For this review, take the finished solid that the model builds, in its own axes (mm). A direction names the side the tool comes from. Coordinates: 2 decimals unless noted, no trailing zeros. Write each loop counter-clockwise with the first axis right and the second up, starting at its lowest first coordinate (ties: lowest second). Pieces come first, ordered by that corner, then holes. Notation, with made-up numbers: M -0.75,12 L 26.25,12 A17 cw 26.25,26 Z; hole C -32,53.25 d2. An arc over 180 degrees is marked long. Return JSON: item names as keys, results as strings.
```python
from build123d import *
from build123d.topology import SkipClean

# Parameters (mm, degrees)
BOSS_EXTRUDE1_DEPTH = 2.032
SKETCH2_R           = 3.81
SKETCH2_R_2         = 1.143
CUT_EXTRUDE1_DEPTH  = 13.861532724
BOSS_EXTRUDE2_START = 9.652
SKETCH3_R           = 7.62
SKETCH3_R_2         = 6.82
BOSS_EXTRUDE2_DEPTH = 9.652
SKETCH4_W           = 25.828848912
SKETCH4_H           = 4.572
CUT_EXTRUDE2_DEPTH  = 16.951523564
BOSS_EXTRUDE3_START = 11.43
SKETCH5_R           = 6.82
BOSS_EXTRUDE3_DEPTH = 11.43


with BuildPart() as part:
    # Sketch1 → Boss-Extrude1 (new body)
    with BuildSketch(Plane(origin=(0, 0, 0), x_dir=(1, 0, 0), z_dir=(0, 1, 0))):
        with BuildLine():
            ThreePointArc((-6.530513036, -3.926423243), (0, -7.62), (6.530513036, -3.926423243))
            ThreePointArc((6.530513036, -3.926423243), (7.220592933, -3.152220394), (8.145517241, -2.683055883))
            ThreePointArc((8.145517241, -2.683055883), (10.16, 0), (8.145517241, 2.683055883))
            ThreePointArc((8.145517241, 2.683055883), (7.220592933, 3.152220394), (6.530513036, 3.926423243))
            ThreePointArc((6.530513036, 3.926423243), (0, 7.62), (-6.530513036, 3.926423243))
            ThreePointArc((-6.530513036, 3.926423243), (-7.220592933, 3.152220394), (-8.145517241, 2.683055883))
            ThreePointArc((-8.145517241, 2.683055883), (-10.16, 0), (-8.145517241, -2.683055883))
            ThreePointArc((-8.145517241, -2.683055883), (-7.220592933, -3.152220394), (-6.530513036, -3.926423243))
        make_face()
    extrude(amount=BOSS_EXTRUDE1_DEPTH)

    # Sketch2 → Cut-Extrude1 (cut, through all)
    with BuildSketch(Plane(origin=(0, 2.032, 0), x_dir=(1, 0, 0), z_dir=(0, 1, 0))):
        with Locations(Location((0, 0, 0), (0, 0, 270))):
            Circle(SKETCH2_R)
        with Locations(Location((-7.366, 0, 0), (0, 0, 270))):
            Circle(SKETCH2_R_2)
        with Locations(Location((7.366, 0, 0), (0, 0, 270))):
            Circle(SKETCH2_R_2)
    extrude(amount=-CUT_EXTRUDE1_DEPTH, mode=Mode.SUBTRACT)

    # Sketch3 → Boss-Extrude2 (add)
    with SkipClean():  # the faces are left unmerged after this step: merging them gives an invalid solid
        with BuildSketch(Plane.XZ.offset(BOSS_EXTRUDE2_START)):
            with Locations(Location((0, 0, 0), (0, 0, 270))):
                Circle(SKETCH3_R)
            with Locations(Location((0, 0, 0), (0, 0, 171.875802718))):
                Circle(SKETCH3_R_2, mode=Mode.SUBTRACT)
        extrude(amount=-BOSS_EXTRUDE2_DEPTH)

    # Sketch4 → Cut-Extrude2 (cut, through all)
    with SkipClean():  # the faces are left unmerged after this step: merging them gives an invalid solid
        with BuildSketch(Plane.XZ):
            Rectangle(SKETCH4_W, SKETCH4_H)
        extrude(amount=CUT_EXTRUDE2_DEPTH, mode=Mode.SUBTRACT)

    # Sketch5 → Boss-Extrude3 (add)
    with SkipClean():  # the faces are left unmerged after this step: merging them gives an invalid solid
        with BuildSketch(Plane.XZ.offset(BOSS_EXTRUDE3_START)):
            with Locations(Location((0, 0, 0), (0, 0, 160.415870392))):
                Circle(SKETCH5_R)
        extrude(amount=-BOSS_EXTRUDE3_DEPTH)


solid = part.part
```
1. Clearance check with flat-ended pins moving along their axes: pin 1 Ø1 at (x, y) = (5, -3.5) entering from -Z; pin 2 Ø2 at (y, z) = (-9.5, -4) entering from +X; pin 3 Ø8 at (y, z) = (0.5, 5) entering from +X. State where each tip first meets the part, or that it passes through.
Checks:
{"pin 1": "z = -6.15", "pin 2": "x = 7", "pin 3": "x = 9.97"}
2. Draft analysis for pull direction X (two halves, no side actions). For faces 1 (the face through (-0.14, -3.89, -7.62)), 2 (the face through (6.25, 1.03, -0.25)), 3 (the face through (7, -5, 2.286)), 4 (the face through (3.778, 1.03, -0.496)), state which applies: +X half, -X half, draft (parallel to the pull), parting line (faces both ways), or undercut.
Checks:
{"face 1": "parting line", "face 2": "undercut", "face 3": "draft", "face 4": "undercut"}
3. We need section C-C (y = -5). State the section outline as (x, z) points.
Checks:
{"outline": "M -7.27,-2.29 A7.62 ccw 7.27,-2.29 L 6.43,-2.29 A6.82 ccw 6.43,2.29 L 7.27,2.29 A7.62 ccw -7.27,2.29 L -6.43,2.29 A6.82 ccw -6.43,-2.29 Z"}
4. We need section D-D (z = -3). State the section outline as (x, y) points.
Checks:
{"outline": "M -7.44,0 L -7,0 L -7,-9.65 L -6.12,-9.65 L -6.12,-11.43 L 6.12,-11.43 L 6.12,-9.65 L 7,-9.65 L 7,0 L 7.44,0 L 7.44,2.03 L 2.35,2.03 L 2.35,0 L -2.35,0 L -2.35,2.03 L -7.44,2.03 Z"}
5. We need section A-A (x = 0). State the section outline as (y, z) points, plus the area to 3 significant figures.
Checks:
{"outline": "M -11.43,-6.82 L -9.65,-6.82 L -9.65,-7.62 L 2.03,-7.62 L 2.03,-3.81 L 0,-3.81 L 0,3.81 L 2.03,3.81 L 2.03,7.62 L -9.65,7.62 L -9.65,6.82 L -11.43,6.82 Z", "area": "187 mm2"}
6. We need section B-B (z = 0). State the section outline as (x, y) points, plus the area to 3 significant figures.
Checks:
{"outline": "M -10.16,0 L -8.51,0 L -8.51,2.03 L -10.16,2.03 Z; M -6.82,-11.43 L 6.82,-11.43 L 6.82,0 L 6.22,0 L 6.22,2.03 L 3.81,2.03 L 3.81,0 L -3.81,0 L -3.81,2.03 L -6.22,2.03 L -6.22,0 L -6.82,0 Z; M 8.51,0 L 10.16,0 L 10.16,2.03 L 8.51,2.03 Z", "area": "172 mm2"}
7. For faces 5 (the face through (-7, -5, -2.286)), 6 (the face through (-6.4, 1.03, 0.61)), 7 (the face through (-1, -9.652, -7)), 8 (the face through (7, -5, -2.286)), 9 (the face through (0, -9.652, 7)), list the 3-axis set-ups (+Z, -Z, +X, -X, +Y, -Y) from which the entire face can be reached by the end or side of a thin tool; tool diameter is ignored.
Checks:
{"face 5": "-X, -Y", "face 6": "+Y", "face 7": "-Z, -Y", "face 8": "+X, -Y", "face 9": "+Z, -Y"}
8. Wall thickness on L1, parallel to X at y = 1.15, z = 0; L2, parallel to Z at x = 0, y = 1.15; L3, parallel to Y at x = -7.5, z = 1.5: over which ranges is each line inside the solid? List them lowest first. Write a range as from..to.
Checks:
{"L1": "-10.16..-8.51, -6.22..-3.81, 3.81..6.22, 8.51..10.16", "L2": "-7.62..-3.81, 3.81..7.62", "L3": "0..2.03"}
